CAD build for the part. Positions are in the model's coordinates, mm. Round coordinates to 2 decimals unless told otherwise and drop trailing zeros. Loops run counter-clockwise (first coordinate to the right, second up) from the corner with the lowest first, then second, coordinate; pieces in that order, holes last. Notation, with made-up numbers: (85.25, 1.25) - (107.25, 1.25) arc R22 ccw to (107.25, 10.25) - close; hole circle Ø6 at (-26, -29.75). An arc over 180 degrees is marked (long way). One line per question, with ' | ' between items.
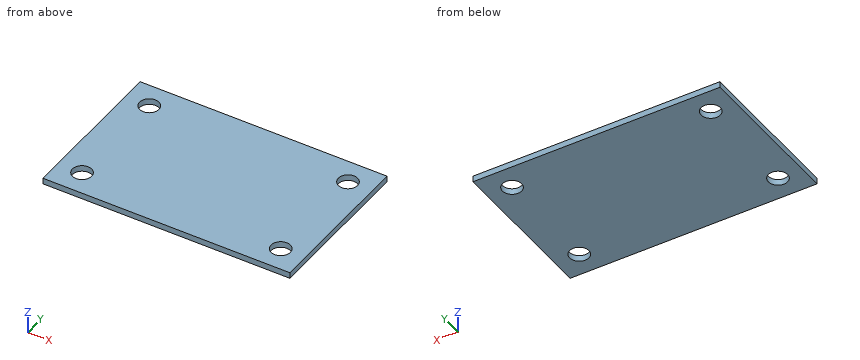
Solid Edge part; units mm, degrees
sketch "Sketch1" plane through (0, 0, 0) normal (0, 0, 1) x (1, 0, 0)
  line L0 (-20.5, -13) -> (20.5, -13)
  line L1 (20.5, -13) -> (20.5, 13)
  line L2 (20.5, 13) -> (-20.5, 13)
  line L3 (-20.5, 13) -> (-20.5, -13)
  dimension "D1" = 20.5
  dimension "D2" = 20.5
extrude "Protrusion1" add sketch "Sketch1" along normal blind 1
hole "Hole_1" at (-16.5, 9, 1) direction (0, 0, -1) diameter 3.2 end up to next
hole "Hole1" at (16.5, 9, 1) direction (0, 0, -1) diameter 3.2 end up to next
hole "Hole2" at (16.5, -9, 1) direction (0, 0, -1) diameter 3.2 end up to next
hole "Hole3" at (-16.5, -9, 1) direction (0, 0, -1) diameter 3.2 end up to next
properties material "Polyethylene, low density"
(1) Cut at C-C, the plane z = 0.35. Write the cut outline in (x, y).
Results found:
outline: (-20.5, -13) - (20.5, -13) - (20.5, 13) - (-20.5, 13) - close; hole circle Ø3.2 at (-16.5, -9); hole circle Ø3.2 at (-16.5, 9); hole circle Ø3.2 at (16.5, -9); hole circle Ø3.2 at (16.5, 9)
(2) Probe L1, parallel to X at y = -9, z = 0.5; L2, parallel to Y at x = -16.5, z = 0.6; L3, parallel to X at y = -8.25, z = 0.4. List the from-to ranges inside material, lowest first.
Results found:
L1: x = -20.5 to -18.1, -14.9 to 14.9, 18.1 to 20.5 | L2: y = -13 to -10.6, -7.4 to 7.4, 10.6 to 13 | L3: x = -20.5 to -17.91, -15.09 to 15.09, 17.91 to 20.5
(3) Cut at B-B, the plane x = 16.5. Write the cut outline in (y, z), then the cut area to 3 significant figures.
Results found:
outline: (-13, 0) - (-10.6, 0) - (-10.6, 1) - (-13, 1) - close; (-7.4, 0) - (7.4, 0) - (7.4, 1) - (-7.4, 1) - close; (10.6, 0) - (13, 0) - (13, 1) - (10.6, 1) - close | area: 19.6 mm²
(4) Drop flat-ended pins along their axis: P1, Ø3.5, axis at x = 16.5, y = 9, coming from the -Z side; P2, Ø3, axis at x = -16.5, y = 9, coming from the +Z side (3 decimals). Give the stop position or say it passes through.
Results found:
P1: stops at z = 0 | P2: passes through
(5) Cut at A-A, the plane y = 9. Write the cut outline in (x, z).
Results found:
outline: (-20.5, 0) - (-18.1, 0) - (-18.1, 1) - (-20.5, 1) - close; (-14.9, 0) - (14.9, 0) - (14.9, 1) - (-14.9, 1) - close; (18.1, 0) - (20.5, 0) - (20.5, 1) - (18.1, 1) - close
